The model under review builds one solid part; all positions refer to its coordinate system, in mm. A direction names the side the tool comes from. Coordinates: 2 decimals unless noted, no trailing zeros. Write each loop counter-clockwise with the first axis right and the second up, starting at its lowest first coordinate (ties: lowest second). Pieces come first, ordered by that corner, then holes.
1) For P1, Ø2, axis at x = 11, y = 4, coming from the +Z side; P2, Ø1.5, axis at y = 8, z = -59.5, coming from the +X side; P3, Ø10, axis at y = -3, z = 40.5, coming from the -X side; P4, Ø3, axis at y = 9, z = 16, coming from the -X side, all flat-tipped, find the tip position at first contact; note any pin that passes through.
2) Machinability: for faces 1 (the flat face through (3, 6.35, -1)), 2 (the flat face through (8, -12.7, -2)), which of the approach directions +Z, -Z, +X, -X, +Y, -Y give a long, thin tool a straight path to every point of the face, cutting with its end or side? Answer none if there is none.
3) For line 1 (Y direction, x = 4.5, z = -24); line 2 (X direction, y = -5.5, z = 74); line 3 (Z direction, x = 10.25, y = -11.25), list the stretches that pass through material, from the lowest coordinate up.
4) Add section B-B, the plane x = 2. State the section outline as (y, z) points.
5) Add section A-A, the plane z = 42. State the section outline as (x, y) points (3 decimals).
6) Add section C-C, the plane y = -2.75. State the section outline as (x, z) points.
from build123d import *

# Parameters (mm, degrees)
F0_W     = 25.4
F0_H     = 215.9
F1_DEPTH = 15.875
F3_W     = 6.35
F3_H     = 6.35
F4_DEPTH = 215.901
F5_DEPTH = 15.876
F6_SIZE2 = 19.0554861232
F6_SIZE  = 6.35


with BuildPart() as f1:
    # F0 (on Right) → F1 (new body)
    with BuildSketch(Plane.YZ):
        Rectangle(F0_W, F0_H)
    extrude(amount=F1_DEPTH)

    # F3 (on face) → F4 (cut, through all)
    with BuildSketch(Plane(origin=(0, 0, -107.95), x_dir=(1, 0, 0), z_dir=(0, 0, -1))):
        with Locations((3.175, -9.525)):
            Rectangle(F3_W, F3_H)
    extrude(amount=-F4_DEPTH, mode=Mode.SUBTRACT)

    # F2 (on face) → F5 (cut, through all)
    with BuildSketch(Plane.YZ.offset(15.875)):
        Polygon((12.7, 107.95), (-12.7, 107.95), (12.7, 82.55), align=None)
        Polygon((12.7, -82.55), (-12.7, -107.95), (12.7, -107.95), align=None)
    extrude(amount=-F5_DEPTH, mode=Mode.SUBTRACT)

    # F6
    f6_edges = [f1.edges().sort_by_distance(p)[0] for p in [
        (15.875, 12.7, 0),
    ]]
    f6_side = f1.faces().sort_by_distance((11.1125, 12.7, 0))[0]
    chamfer(f6_edges, length=F6_SIZE, length2=F6_SIZE2, reference=f6_side)


solid = f1.part
Geometry results:
1. P1: stops at z = 92.25
1. P2: stops at x = 11.34
1. P3: stops at x = 0
1. P4: stops at x = 6.35
2. face 1: +Z, -Z, -X, +Y
2. face 2: +Z, -Z, +X, -X, -Y
3. line 1: y = -12.7 to 6.35
3. line 2: x = 0 to 15.59
3. line 3: z = -106.5 to 106.5
4. outline: (-12.7, -107.95) - (6.35, -88.9) - (6.35, 88.9) - (-12.7, 107.95) - close
5. outline: (0, -12.7) - (15.875, -12.7) - (15.875, -6.355) - (9.525, 12.7) - (6.35, 12.7) - (6.35, 6.35) - (0, 6.35) - close
6. outline: (0, -98) - (14.67, -98) - (14.67, 98) - (0, 98) - close
